from build123d import *

# Parameters (mm, degrees)
SKETCH_1_W          = 42
SKETCH_1_H          = 56
EXTRUDE_1_DEPTH     = 5
SKETCH_2_W          = 5
SKETCH_2_H          = 56
EXTRUDE_2_DEPTH     = 23
SKETCH_3_W          = 3
SKETCH_3_H          = 7.5
EXTRUDE_3_DEPTH     = 20.2
SKETCH_4_R          = 1.75
CUT_EXTRUDE_1_DEPTH = 36.7
SKETCH_5_R          = 1.65
CUT_EXTRUDE_2_DEPTH = 10


with BuildPart() as part:
    # 草图1 → 凸台-拉伸1 (new body)
    with BuildSketch(Plane.XY):
        Rectangle(SKETCH_1_W, SKETCH_1_H)
    extrude(amount=EXTRUDE_1_DEPTH)

    # 草图2 → 凸台-拉伸2 (add)
    with BuildSketch(Plane.XY.offset(5)):
        with Locations((-23.5, 0)):
            Rectangle(SKETCH_2_W, SKETCH_2_H)
    extrude(amount=-EXTRUDE_2_DEPTH)

    # 草图3 → 凸台-拉伸3 (add)
    with BuildSketch(Plane(origin=(0, 0, 0), x_dir=(-1, 0, 0), z_dir=(0, 0, -1))):
        with Locations((-8.2, -24.25)):
            Rectangle(SKETCH_3_W, SKETCH_3_H)
        with Locations((-8.2, 24.25)):
            Rectangle(SKETCH_3_W, SKETCH_3_H)
    extrude(amount=EXTRUDE_3_DEPTH)

    # 草图4 → 切除-拉伸1 (cut, through all)
    with BuildSketch(Plane(origin=(9.7, 0, 0), x_dir=(0, 0, -1), z_dir=(1, 0, 0))):
        with Locations((5.1, 24.25)):
            Circle(SKETCH_4_R)
        with Locations((15.1, 24.25)):
            Circle(SKETCH_4_R)
        with Locations((15.1, -24.25)):
            Circle(SKETCH_4_R)
        with Locations((5.1, -24.25)):
            Circle(SKETCH_4_R)
    extrude(amount=-CUT_EXTRUDE_1_DEPTH, mode=Mode.SUBTRACT)

    # 草图5 → 切除-拉伸2 (cut)
    with BuildSketch(Plane(origin=(0, 0, 0), x_dir=(-1, 0, 0), z_dir=(0, 0, -1))):
        with Locations((-16, 23)):
            Circle(SKETCH_5_R)
        with Locations((-16, -23)):
            Circle(SKETCH_5_R)
        with Locations((16, -23)):
            Circle(SKETCH_5_R)
        with Locations((16, 23)):
            Circle(SKETCH_5_R)
        with Locations((16, 0)):
            Circle(SKETCH_5_R)
        with Locations((-16, 0)):
            Circle(SKETCH_5_R)
    extrude(amount=-CUT_EXTRUDE_2_DEPTH, mode=Mode.SUBTRACT)


solid = part.part
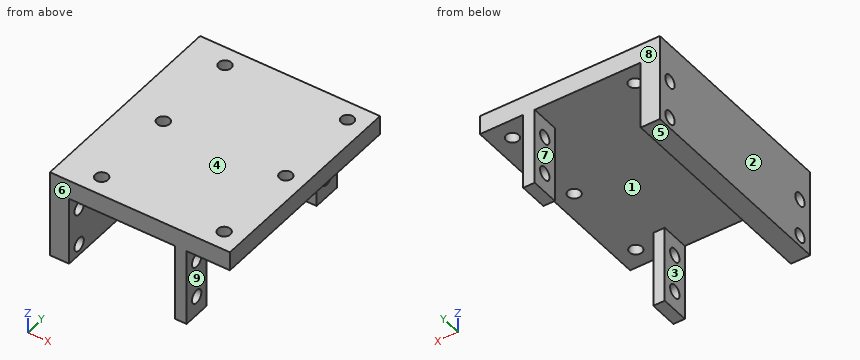
Geometry check sheet. Reference: the model listing, model coordinates, mm. Face numbers are marked on the shaded views. A direction names the side the tool comes from. Give positions to 0.01 mm unless a question says otherwise; leave off trailing zeros. Loops run counter-clockwise (first coordinate to the right, second up) from the corner with the lowest first, then second, coordinate; pieces in that order, holes last. Notation, with made-up numbers: M -10,60.25 L 16,60.25 A18 ccw 16,89.25 Z; hole C 56.25,5 d8. An arc over 180 degrees is marked long. Write each question's results on one line, items separated by ' | '.
1) Release check for a two-part mould opening along X. For the marked faces 1, 2, 3 and 4 record: +X half, -X half, draft (parallel to the pull), parting line (faces both ways), or undercut.
Answers follow:
face 1: undercut | face 2: -X half | face 3: undercut | face 4: draft
2) Section check A-A, the plane x = 16. Record the boundary of the cut face in (y, z).
Answers follow:
outline: M -28,0 L -24.65,0 L -24.65,5 L -28,5 Z; M -21.35,0 L -1.65,0 L -1.65,5 L -21.35,5 Z; M 1.65,0 L 21.35,0 L 21.35,5 L 1.65,5 Z; M 24.65,0 L 28,0 L 28,5 L 24.65,5 Z
3) Thickness scan on line 1 (Y direction, x = -16, z = 3.2); line 2 (Y direction, x = -23.7, z = -5.1); line 3 (Z direction, x = -23, y = -24). Record the ranges inside material, lowest first.
Answers follow:
line 1: -28 to -24.65, -21.35 to -1.65, 1.65 to 21.35, 24.65 to 28 | line 2: -28 to -26, -22.5 to 22.5, 26 to 28 | line 3: -18 to -16.83, -13.37 to -6.83, -3.37 to 5
4) Section check B-B, the plane z = -15.1. Record the boundary of the cut face in (x, y), plus the area to 3 significant figures.
Answers follow:
outline: M -26,-28 L -21,-28 L -21,-26 L -26,-26 Z; M -26,-22.5 L -21,-22.5 L -21,22.5 L -26,22.5 Z; M -26,26 L -21,26 L -21,28 L -26,28 Z; M 6.7,-28 L 9.7,-28 L 9.7,-26 L 6.7,-26 Z; M 6.7,-22.5 L 9.7,-22.5 L 9.7,-20.5 L 6.7,-20.5 Z; M 6.7,20.5 L 9.7,20.5 L 9.7,22.5 L 6.7,22.5 Z; M 6.7,26 L 9.7,26 L 9.7,28 L 6.7,28 Z | area: 269 mm2
5) Gauge pin test, flat ends, axial feed: pin 1 (4 mm diameter, centred on y = -24.25, z = -5.1, fed in from +X); pin 2 (5.5 mm diameter, centred on x = 16, y = -23, fed in from -Z); pin 3 (2.5 mm diameter, centred on x = -24.5, y = -13.5, fed in from -Z). Record the tip position at first contact, or that the pin passes through.
Answers follow:
pin 1: x = 9.7 | pin 2: z = 0 | pin 3: z = -18
6) Section check C-C, the plane z = -8.75. Record the boundary of the cut face in (x, y).
Answers follow:
outline: M -26,-28 L -21,-28 L -21,28 L -26,28 Z; M 6.7,-28 L 9.7,-28 L 9.7,-20.5 L 6.7,-20.5 Z; M 6.7,20.5 L 9.7,20.5 L 9.7,28 L 6.7,28 Z
7) Tool access check on the marked faces 5, 6, 7, 8 and 9. Record the directions out of +Z, -Z, +X, -X, +Y, -Y that give a thin tool (end or side, any length) a straight path to the whole face; none if there is none.
Answers follow:
face 5: -Z, -X, +Y, -Y | face 6: +Z, -Z, +X, -X, -Y | face 7: -Z, +Y, -Y | face 8: +Z, -Z, +X, -X, +Y | face 9: -Z, +X, +Y, -Y
8) Section check D-D, the plane y = 0. Record the boundary of the cut face in (x, z).
Answers follow:
outline: M -26,-18 L -21,-18 L -21,0 L -17.65,0 L -17.65,5 L -26,5 Z; M -14.35,0 L 14.35,0 L 14.35,5 L -14.35,5 Z; M 17.65,0 L 21,0 L 21,5 L 17.65,5 Z
